Can you work these out from the model? Positions are in its coordinate system, mm. A direction names the side the tool comes from. Give positions to 0.01 mm unless a question says otherwise; leave off trailing zeros. Write each loop counter-clockwise with the first axis right and the second up, starting at its lowest first coordinate (ties: lowest second). Pieces come first, ordered by that corner, then holes.
```python
from build123d import *

# Parameters (mm, degrees)
SKETCH1_W           = 25.4
SKETCH1_H           = 25.4
BOSS_EXTRUDE1_DEPTH = 114.3
SKETCH2_W           = 19.05
SKETCH2_H           = 19.05
CUT_EXTRUDE1_DEPTH  = 116.702506455
SKETCH3_R           = 3.2639
CUT_EXTRUDE2_DEPTH  = 118.774954893


with BuildPart() as part:
    # Sketch1 → Boss-Extrude1 (new body)
    with BuildSketch(Plane.XY):
        Rectangle(SKETCH1_W, SKETCH1_H)
    extrude(amount=BOSS_EXTRUDE1_DEPTH)

    # Sketch2 → Cut-Extrude1 (cut, through all)
    with BuildSketch(Plane.XY):
        Rectangle(SKETCH2_W, SKETCH2_H)
    extrude(amount=CUT_EXTRUDE1_DEPTH, mode=Mode.SUBTRACT)

    # Sketch3 → Cut-Extrude2 (cut, through all)
    with BuildSketch(Plane(origin=(0, 12.7, 0), x_dir=(1, 0, 0), z_dir=(0, 1, 0))):
        with Locations(Location((0, -99.314, 0), (0, 0, 180))):
            Circle(SKETCH3_R)
    extrude(amount=-CUT_EXTRUDE2_DEPTH, mode=Mode.SUBTRACT)


solid = part.part
```
1) For faces 4 (the face through (-9.525, 0, 56)), 5 (the face through (-12.7, 0, 56)), which set-ups out of +Z, -Z, +X, -X, +Y, -Y let a thin tool reach every point of the face, with its end or its side?
Values follow:
face 4: +Z, -Z
face 5: +Z, -Z, -X, +Y, -Y
2) Suppose I cut it at A-A on z = 38. Write out the boundary of the cut face in (x, y) (3 decimals).
Values follow:
outline: (-12.7, -12.7) - (12.7, -12.7) - (12.7, 12.7) - (-12.7, 12.7) - close; hole (-9.525, -9.525) - (9.525, -9.525) - (9.525, 9.525) - (-9.525, 9.525) - close
3) If we mould it in two halves opening along X, with no side actions, what happens to faces 1 (the face through (9.525, 0, 56)), 2 (the face through (0, 12.7, 56)), 3 (the face through (12.7, 0, 56))? For each: +X half, -X half, draft (parallel to the pull), parting line (faces both ways), or undercut.
Values follow:
face 1: undercut
face 2: draft
face 3: +X half
4) Please list where these lines run through material, in increasing order: L1, parallel to X at y = 7, z = 77.5 (3 decimals); L2, parallel to Z at x = 0, y = -10.9.
Values follow:
L1: x = -12.7 to -9.525, 9.525 to 12.7
L2: z = 0 to 96.05, 102.58 to 114.3
5) Suppose I cut it at C-C on x = 0. Write out the boundary of the cut face in (y, z) (3 decimals).
Values follow:
outline: (-12.7, 0) - (-9.525, 0) - (-9.525, 96.05) - (-12.7, 96.05) - close; (-12.7, 102.578) - (-9.525, 102.578) - (-9.525, 114.3) - (-12.7, 114.3) - close; (9.525, 0) - (12.7, 0) - (12.7, 96.05) - (9.525, 96.05) - close; (9.525, 102.578) - (12.7, 102.578) - (12.7, 114.3) - (9.525, 114.3) - close
6) Suppose I cut it at B-B on x = 5. Write out the boundary of the cut face in (y, z) (3 decimals), plus the area to 3 significant figures.
Values follow:
outline: (-12.7, 0) - (-9.525, 0) - (-9.525, 114.3) - (-12.7, 114.3) - close; (9.525, 0) - (12.7, 0) - (12.7, 114.3) - (9.525, 114.3) - close
area: 726 mm2
7) For pin 1 Ø2 at (x, y) = (3.5, -9.5) entering from +Z; pin 2 Ø6 at (x, z) = (0, 99.314) entering from -Y, each with a flat end and sliding along its axis, tell me the tip position at first contact or that it passes through.
Values follow:
pin 1: stops at z = 114.3
pin 2: passes through
